from build123d import *

# Parameters (mm, degrees)
DODANIE_WYCI_GNI_CIE1_DEPTH = 46


with BuildPart() as part:
    # Szkic1 → Dodanie-wyciągnięcie1 (new body)
    with BuildSketch(Plane.XY):
        with BuildLine():
            Line((0, 0), (8.237634002, 0))
            Line((8.237634002, 0), (37.237634002, 36))
            Line((37.237634002, 36), (37.237634002, 56.863352311))
            Line((37.237634002, 56.863352311), (33.343864456, 60))
            Line((33.343864456, 60), (4.343864456, 60))
            ThreePointArc((4.343864456, 60), (-2.880934736, 56.327791154), (-10.978818754, 56.000505938))
            Line((-10.978818754, 56.000505938), (-38.762365998, 60.899494937))
            Line((-38.762365998, 60.899494937), (-47.81261853, 60.899494937))
            Line((-47.81261853, 60.899494937), (-52.762365998, 55.949747468))
            Line((-52.762365998, 55.949747468), (-52.762365998, 23.949747468))
            Line((-52.762365998, 23.949747468), (-47.81261853, 19))
            Line((-47.81261853, 19), (-11.02625203, 19))
            ThreePointArc((-11.02625203, 19), (-7.70519621, 17.737725008), (-6.060974673, 14.588235294))
            ThreePointArc((-6.060974673, 14.588235294), (-4.04296027, 6.873465479), (0, 0))
        make_face()
    extrude(amount=DODANIE_WYCI_GNI_CIE1_DEPTH)


solid = part.part
Model file for the job. Use its own axes, mm. A direction names the side the tool comes from. Coordinates: 2 decimals unless noted, no trailing zeros. Order: outer loops, then holes, each group sorted by start corner. A loop starts at its lowest first (then second) coordinate and runs counter-clockwise, first axis right, second up. Notation, with made-up numbers: (51.5, 2.5) -> (61.5, 2.5) arc R15 cw to (61.5, 30.5) -> close; hole circle Ø3 at (15, -11). An arc over 180 degrees is marked (long way). Return JSON: item names as keys, results as strings. Group by question number.
Item 1: Saw through at B-B on x = -14. Write the cut outline in (y, z).
Item 2: Wall check: line 1 along Y through (x, z) = (-47.5, 5); line 2 along Y through (x, z) = (8, 33.5); line 3 along X through (y, z) = (13, 44). Give the ranges that are in metal, low to high. Write a range as [from, to].
Item 3: Tool access for faces 1 (the flat face through (-30, 19, 23)), 2 (the flat face through (-43, 60.899, 23)), 3 (the flat face through (19, 60, 23)), 4 (the flat face through (-24.676, 58.416, 22.678)): list every direction of +Z, -Z, +X, -X, +Y, -Y with a clear straight run to the whole face (end or side of a thin tool).
Item 4: Saw through at C-C on y = 11. Write the cut outline in (x, z).
Item 5: Flat gauge pins, fed straight in: P1, Ø1.5, axis at y = 8.5, z = 21, coming from the -X side; P2, Ø1, axis at x = 5.5, z = 32.5, coming from the +Y side; P3, Ø4, axis at y = 27, z = 39.5, coming from the +X side. Where does each tip first touch, or does it go through?
Item 6: Saw through at A-A on z = 28.5. Write the cut outline in (x, y).
Values found:
{
 "1": {"outline": "(19, 0) -> (56.53, 0) -> (56.53, 46) -> (19, 46) -> close"},
 "2": {"line 1": "y = [19, 60.9]", "line 2": "y = [0, 60]", "line 3": "x = [-5.83, 18.71]"},
 "3": {"face 1": "+Z, -Z, -X, -Y", "face 2": "+Z, -Z, +X, -X, +Y", "face 3": "+Z, -Z, +X, +Y", "face 4": "+Z, -Z, +Y"},
 "4": {"outline": "(-5.4, 0) -> (17.1, 0) -> (17.1, 46) -> (-5.4, 46) -> close"},
 "5": {"P1": "stops at x = -4.91", "P2": "stops at y = 60", "P3": "stops at x = 31.6"},
 "6": {"outline": "(-52.76, 23.95) -> (-47.81, 19) -> (-11.03, 19) arc R5 cw to (-6.06, 14.59) arc R29 ccw to (0, 0) -> (8.24, 0) -> (37.24, 36) -> (37.24, 56.86) -> (33.34, 60) -> (4.34, 60) arc R19 cw to (-10.98, 56) -> (-38.76, 60.9) -> (-47.81, 60.9) -> (-52.76, 55.95) -> close"}
}
